from build123d import *

# Parameters (mm, degrees)
SKETCH1_W           = 50
SKETCH1_H           = 50
BOSS_EXTRUDE1_DEPTH = 4
SKETCH2_R           = 4.1
CUT_EXTRUDE1_DEPTH  = 4
SKETCH5_R           = 10
SKETCH5_R_2         = 4.1
BOSS_EXTRUDE4_DEPTH = 2.6
SKETCH6_OUTSIDE_W   = 66.204
SKETCH6_OUTSIDE_H   = 66.204
CUT_EXTRUDE3_DEPTH  = 4
SKETCH7_W           = 29
SKETCH7_H           = 4
BOSS_EXTRUDE5_DEPTH = 30
SKETCH8_R           = 1.55
CUT_EXTRUDE4_DEPTH  = 4
CUT_EXTRUDE5_DEPTH  = 2


with BuildPart() as part:
    # Sketch1 → Boss-Extrude1 (new body)
    with BuildSketch(Plane(origin=(0, 0, 0), x_dir=(1, 0, 0), z_dir=(0, 1, 0))):
        with Locations((-21.122518296, -46.495755178)):
            Rectangle(SKETCH1_W, SKETCH1_H)
    extrude(amount=BOSS_EXTRUDE1_DEPTH)

    # Sketch2 → Cut-Extrude1 (cut)
    with BuildSketch(Plane.XZ):
        with Locations(Location((-21.122518296, 46.495755178, 0), (0, 0, 270))):
            Circle(SKETCH2_R)
    extrude(amount=-CUT_EXTRUDE1_DEPTH, mode=Mode.SUBTRACT)

    # Sketch5 → Boss-Extrude4 (add)
    with BuildSketch(Plane(origin=(0, 4, 0), x_dir=(1, 0, 0), z_dir=(0, 1, 0))):
        with Locations(Location((-21.122518296, -46.495755178, 0), (0, 0, 270))):
            Circle(SKETCH5_R)
        with Locations(Location((-21.122518296, -46.495755178, 0), (0, 0, 90))):
            Circle(SKETCH5_R_2, mode=Mode.SUBTRACT)
    extrude(amount=BOSS_EXTRUDE4_DEPTH)

    # Sketch6 outside → Cut-Extrude3 (cut)
    with BuildSketch(Plane.XZ):
        with Locations((-21.123, 46.496)):
            Rectangle(SKETCH6_OUTSIDE_W, SKETCH6_OUTSIDE_H)
        with BuildLine():
            Line((-35.622518296, 46.495755178), (-35.622518296, 21.495755178))
            Line((-35.622518296, 21.495755178), (-6.622518296, 21.495755178))
            Line((-6.622518296, 21.495755178), (-6.622518296, 46.495755178))
            ThreePointArc((-6.622518296, 46.495755178), (-21.122518296, 60.995755178), (-35.622518296, 46.495755178))
        make_face(mode=Mode.SUBTRACT)
    extrude(amount=-CUT_EXTRUDE3_DEPTH, mode=Mode.SUBTRACT)

    # Sketch7 → Boss-Extrude5 (add)
    with BuildSketch(Plane(origin=(0, 0, 21.495755178), x_dir=(-1, 0, 0), z_dir=(0, 0, -1))):
        with Locations((21.122518296, 2)):
            Rectangle(SKETCH7_W, SKETCH7_H)
    extrude(amount=BOSS_EXTRUDE5_DEPTH)

    # Sketch8 → Cut-Extrude4 (cut)
    with BuildSketch(Plane(origin=(0, 4, 0), x_dir=(1, 0, 0), z_dir=(0, 1, 0))):
        with Locations(Location((-26.779372546, -0.338900928, 0), (0, 0, 270))):
            Circle(SKETCH8_R)
        with Locations(Location((-15.465664047, -11.652609427, 0), (0, 0, 270))):
            Circle(SKETCH8_R)
    extrude(amount=-CUT_EXTRUDE4_DEPTH, mode=Mode.SUBTRACT)

    # Sketch9 → Cut-Extrude5 (cut)
    with BuildSketch(Plane(origin=(0, 4, 0), x_dir=(1, 0, 0), z_dir=(0, 1, 0))):
        Polygon((-25.047321738, 2.661099072), (-28.511423353, 2.661099072), (-30.243474161, -0.338900928), (-28.511423353, -3.338900928), (-25.047321738, -3.338900928), (-23.315270931, -0.338900928), align=None)
        Polygon((-13.733613239, -8.652609427), (-17.197714854, -8.652609427), (-18.929765662, -11.652609427), (-17.197714854, -14.652609427), (-13.733613239, -14.652609427), (-12.001562432, -11.652609427), align=None)
    extrude(amount=-CUT_EXTRUDE5_DEPTH, mode=Mode.SUBTRACT)


solid = part.part
The listing builds one solid part. Answer for the finished solid, in the listing's coordinates (mm). A direction names the side the tool comes from. Give positions to 0.01 mm unless a question says otherwise; leave off trailing zeros. Order: outer loops, then holes, each group sorted by start corner. A loop starts at its lowest first (then second) coordinate and runs counter-clockwise, first axis right, second up. Notation, with made-up numbers: (75, 79) - (131, 79) arc R21 cw to (131, 106) - close; hole circle Ø8 at (17, 69). An arc over 180 degrees is marked (long way). Answer as CSV lines item,"result".
Q1. A cutting plane is placed at D-D, the plane y = 5.5. Determine the outline of the cut face in (x, z), and give its area (3 significant figures).
Answer key:
outline,"circle Ø20 at (-21.12, 46.5); hole circle Ø8.2 at (-21.12, 46.5)"
area,"261 mm^2"
Q2. Each of these flat-tipped pins is pushed along its axis until it touches: pin 1 Ø3.5 at (x, z) = (-15.47, 11.65) entering from -Y; pin 2 Ø8.5 at (x, z) = (-20, 12.5) entering from +Y; pin 3 Ø6.5 at (x, z) = (-21.12, 46.5) entering from -Y; pin 4 Ø3 at (x, z) = (-27, 1.5) entering from +Y. Where does it stop, or does it pass through?
Answer key:
pin 1,"stops at y = 0"
pin 2,"stops at y = 4"
pin 3,"passes through"
pin 4,"stops at y = 2"
Q3. A cutting plane is placed at B-B, the plane z = 44.5. Determine the outline of the cut face in (x, y), and give its area (3 significant figures).
Answer key:
outline,"(-35.62, 0) - (-24.7, 0) - (-24.7, 6.6) - (-30.92, 6.6) - (-30.92, 4) - (-35.62, 4) - close; (-17.54, 0) - (-6.62, 0) - (-6.62, 4) - (-11.32, 4) - (-11.32, 6.6) - (-17.54, 6.6) - close"
area,"120 mm^2"
Q4. Determine the mould class of faces 1 (the face through (-18.119, 5.282, 56.034)), 2 (the face through (-12.88, 3.014, 13.174)), 3 (the face through (-21, 6.6, 51)) for opening direction X: pulls with the +X half, pulls with the -X half, needs draft (parallel to the pull), parting line crosses it, or undercut.
Answer key:
face 1,"parting line crosses it"
face 2,"undercut"
face 3,"needs draft"
Q5. A cutting plane is placed at C-C, the plane x = -12.75. Determine the outline of the cut face in (y, z).
Answer key:
outline,"(0, -8.5) - (4, -8.5) - (4, 10.36) - (2, 10.36) - (2, 12.95) - (4, 12.95) - (4, 41.03) - (6.6, 41.03) - (6.6, 51.96) - (4, 51.96) - (4, 58.33) - (0, 58.33) - close"
Q6. Straight lines are drawn through the part: L1, parallel to Y at x = -28.25, z = 25; L2, parallel to Z at x = -21.5, y = 5; L3, parallel to Z at x = -12, y = 4.75. For each, find the intervals that lie inside material, in ascending order.
Answer key:
L1,"y = 0 to 4"
L2,"z = 36.5 to 42.41, 50.58 to 56.49"
L3,"z = 42.4 to 50.59"
Q7. A cutting plane is placed at A-A, the plane x = -26. Determine the outline of the cut face in (y, z), and give its area (3 significant figures).
Answer key:
outline,"(0, -8.5) - (4, -8.5) - (4, -2.66) - (2, -2.66) - (2, -1) - (0, -1) - close; (0, 1.68) - (2, 1.68) - (2, 3.34) - (4, 3.34) - (4, 37.77) - (6.6, 37.77) - (6.6, 55.23) - (4, 55.23) - (4, 60.15) - (0, 60.15) - close"
area,"303 mm^2"
Q8. Which of the six approach directions +Z, -Z, +X, -X, +Y, -Y give full straight-line access (tool end or side, diameter ignored) to faces 4 (the face through (-27, 3, 3.339)), 5 (the face through (-21, 2, -8.504))?
Answer key:
face 4,"+Y"
face 5,"-Z, +X, -X, +Y, -Y"
